Here's how the part is built. I have some questions about the finished solid (model axes, mm). Face numbers are marked on the shaded views. A direction names the side the tool comes from. Coordinates: 2 decimals unless noted, no trailing zeros. Write each loop counter-clockwise with the first axis right and the second up, starting at its lowest first coordinate (ties: lowest second). Pieces come first, ordered by that corner, then holes.
(1) Imagine slicing it at D-D, the plane y = 8. List the corners of the cut face in (x, z) for me.
(2) Imagine slicing it at B-B, the plane z = 40. State how many separate pieces and enclosed holes the cut face has, plus the area to 3 significant figures.
(3) Please list where these lines run through material, in increasing order: probe 1 along X at (y, z) = (18.55, 0); probe 2 along X at (y, z) = (17.95, 40); probe 3 along Y at (x, z) = (78, -41.5).
(4) Imagine slicing it at A-A, the plane x = 20.5. List the corners of the cut face in (y, z) for me, plus the area to 3 significant figures.
(5) Which directions (+Z, -Z, +X, -X, +Y, -Y) give clear straight access to the entire face, cutting with the end or side of a thin tool? Please do the marked faces 5 and 6.
(6) Thinking about a two-plate mould opening in Y: for the marked faces 1, 2, 3 and 4, which applies, released by +Y, released by -Y, zero draft, split by the parting line, or undercut?
(7) For pin 1 Ø2.5 at (x, z) = (4, -40) entering from -Y; pin 2 Ø1.9 at (x, z) = (30, -20.5) entering from +Y, each with a flat end and sliding along its axis, tell me the tip position at first contact or that it passes through.
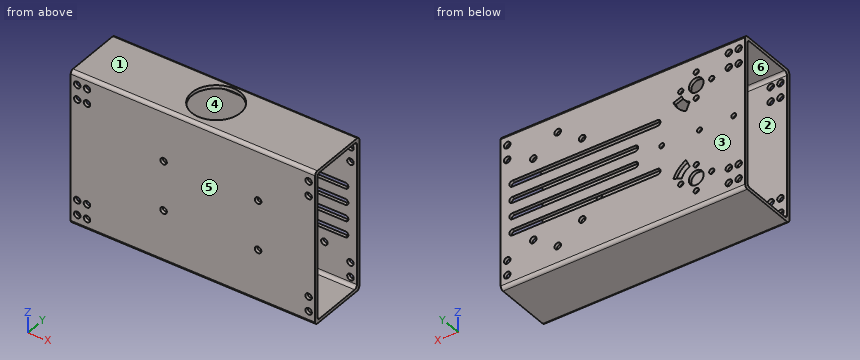
```python
from build123d import *

# Parameters (mm, degrees)
EXTRUDE_1218_DEPTH          = 150
SKETCH_1_R                  = 1.5
SKETCH_1_R_2                = 4.5
SKETCH_1_R_3                = 1.6
CUT_EXTRUDE_1265_DEPTH      = 159.33508771
SKETCH_6_R                  = 15
CUT_EXTRUDE_1532_DEPTH      = 159.33508771
SKETCH_12_R                 = 2
CUT_EXTRUDE_1963_DEPTH      = 2
CUT_EXTRUDE_2327_DEPTH      = 162.260658685
CUT_EXTRUDE_2327_DEPTH_BACK = 162.260658685
SKETCH_14_R                 = 2
SKETCH_15_R                 = 2
CUT_EXTRUDE_2529_DEPTH      = 162.260658685


with BuildPart() as part:
    # 草图2 → Extrude 1218 (new body)
    with BuildSketch(Plane(origin=(0, 0, 0), x_dir=(0, 0, -1), z_dir=(1, 0, 0))):
        with BuildLine():
            Line((-45, 19), (45, 19))
            ThreePointArc((45, 19), (46.414213562, 18.414213562), (47, 17))
            Line((47, 17), (47, -17))
            ThreePointArc((47, -17), (46.414213562, -18.414213562), (45, -19))
            Line((45, -19), (-45, -19))
            ThreePointArc((-45, -19), (-46.414213562, -18.414213562), (-47, -17))
            Line((-47, -17), (-47, 17))
            ThreePointArc((-47, 17), (-46.414213562, 18.414213562), (-45, 19))
        make_face()
        with BuildLine():
            Line((-43, 17), (43, 17))
            ThreePointArc((43, 17), (44.414213562, 16.414213562), (45, 15))
            Line((45, 15), (45, -15))
            ThreePointArc((45, -15), (44.414213562, -16.414213562), (43, -17))
            Line((43, -17), (-43, -17))
            ThreePointArc((-43, -17), (-44.414213562, -16.414213562), (-45, -15))
            Line((-45, -15), (-45, 15))
            ThreePointArc((-45, 15), (-44.414213562, 16.414213562), (-43, 17))
        make_face(mode=Mode.SUBTRACT)
    extrude(amount=EXTRUDE_1218_DEPTH)

    # 草图1 → Cut-Extrude 1265 (cut, through all)
    with BuildSketch(Plane(origin=(0, 0, 0), x_dir=(1, 0, 0), z_dir=(0, 1, 0))):
        with Locations(Location((7, 0, 0), (0, 0, 90))):
            Circle(SKETCH_1_R)
        with Locations(Location((28, 0, 0), (0, 0, 90))):
            Circle(SKETCH_1_R)
        with Locations(Location((51.2, 0, 0), (0, 0, 90))):
            Circle(SKETCH_1_R)
        with Locations(Location((30, -28.5, 0), (0, 0, 90))):
            Circle(SKETCH_1_R_2)
        with Locations(Location((30, 28.5, 0), (0, 0, 90))):
            Circle(SKETCH_1_R_2)
        with Locations(Location((20.5, -28.5, 0), (0, 0, 90))):
            Circle(SKETCH_1_R_3)
        with Locations(Location((39.5, -28.5, 0), (0, 0, 90))):
            Circle(SKETCH_1_R_3)
        with Locations(Location((30, -36.5, 0), (0, 0, 90))):
            Circle(SKETCH_1_R_3)
        with Locations(Location((30, -20.5, 0), (0, 0, 90))):
            Circle(SKETCH_1_R_3)
        with Locations(Location((39.5, 28.5, 0), (0, 0, 90))):
            Circle(SKETCH_1_R_3)
        with Locations(Location((30, 36.5, 0), (0, 0, 90))):
            Circle(SKETCH_1_R_3)
        with Locations(Location((20.5, 28.5, 0), (0, 0, 90))):
            Circle(SKETCH_1_R_3)
        with Locations(Location((30, 20.5, 0), (0, 0, 90))):
            Circle(SKETCH_1_R_3)
        with BuildLine():
            Line((34.014873487, 19.890076023), (36.291936994, 15.006897573))
            ThreePointArc((36.291936994, 15.006897573), (40.941044845, 18.474379532), (43.990135541, 23.40800709))
            Line((43.990135541, 23.40800709), (38.927079897, 25.250808638))
            ThreePointArc((38.927079897, 25.250808638), (37.0041347, 22.081893028), (34.014873487, 19.890076023))
        make_face()
        with BuildLine():
            Line((34.014873487, -19.890076023), (36.291936994, -15.006897573))
            ThreePointArc((36.291936994, -15.006897573), (40.941044845, -18.474379532), (43.990135541, -23.40800709))
            Line((43.990135541, -23.40800709), (38.927079897, -25.250808638))
            ThreePointArc((38.927079897, -25.250808638), (37.0041347, -22.081893028), (34.014873487, -19.890076023))
        make_face()
    extrude(amount=CUT_EXTRUDE_1265_DEPTH, mode=Mode.SUBTRACT)

    # 草图6 → Cut-Extrude 1532 (cut, through all)
    with BuildSketch(Plane.XY):
        with Locations(Location((75, 1, 0), (0, 0, 111.039469781))):
            Circle(SKETCH_6_R)
    extrude(amount=CUT_EXTRUDE_1532_DEPTH, mode=Mode.SUBTRACT)

    # 草图12 → Cut-Extrude 1963 (cut)
    with BuildSketch(Plane(origin=(0, 19, 0), x_dir=(1, 0, 0), z_dir=(0, 1, 0))):
        with Locations(Location((100, 25, 0), (0, 0, 270))):
            Circle(SKETCH_12_R)
        with Locations(Location((130, 25, 0), (0, 0, 270))):
            Circle(SKETCH_12_R)
        with Locations(Location((115, 35, 0), (0, 0, 270))):
            Circle(SKETCH_12_R)
        with Locations(Location((115, -35, 0), (0, 0, 90))):
            Circle(SKETCH_12_R)
        with Locations(Location((130, -25, 0), (0, 0, 90))):
            Circle(SKETCH_12_R)
        with Locations(Location((100, -25, 0), (0, 0, 90))):
            Circle(SKETCH_12_R)
        with BuildLine():
            Line((53.777197841, 16.849529373), (142.85706065, 16.849529373))
            ThreePointArc((142.85706065, 16.849529373), (144.706590023, 15), (142.85706065, 13.150470627))
            Line((142.85706065, 13.150470627), (53.777197841, 13.150470627))
            ThreePointArc((53.777197841, 13.150470627), (51.927668468, 15), (53.777197841, 16.849529373))
        make_face()
        with BuildLine():
            Line((67.529255568, 6.850912176), (142.85706065, 6.850912176))
            ThreePointArc((142.85706065, 6.850912176), (144.707972825, 5), (142.85706065, 3.149087824))
            Line((142.85706065, 3.149087824), (67.529255568, 3.149087824))
            ThreePointArc((67.529255568, 3.149087824), (65.678343393, 5), (67.529255568, 6.850912176))
        make_face()
        with BuildLine():
            Line((53.777197841, -16.849529373), (142.85706065, -16.849529373))
            ThreePointArc((142.85706065, -16.849529373), (144.706590023, -15), (142.85706065, -13.150470627))
            Line((142.85706065, -13.150470627), (53.777197841, -13.150470627))
            ThreePointArc((53.777197841, -13.150470627), (51.927668468, -15), (53.777197841, -16.849529373))
        make_face()
        with BuildLine():
            Line((67.529255568, -6.850912176), (142.85706065, -6.850912176))
            ThreePointArc((142.85706065, -6.850912176), (144.707972825, -5), (142.85706065, -3.149087824))
            Line((142.85706065, -3.149087824), (67.529255568, -3.149087824))
            ThreePointArc((67.529255568, -3.149087824), (65.678343393, -5), (67.529255568, -6.850912176))
        make_face()
    extrude(amount=-CUT_EXTRUDE_1963_DEPTH, mode=Mode.SUBTRACT)

    # 草图14 → Cut-Extrude 2327 (cut, two sides: drawn at the far end of the back side and taken through both)
    with BuildSketch(Plane(origin=(0, -17, 0), x_dir=(1, 0, 0), z_dir=(0, 1, 0)).offset(-CUT_EXTRUDE_2327_DEPTH_BACK)):
        with Locations(Location((4, 40, 0), (0, 0, 270))):
            Circle(SKETCH_14_R)
        with Locations(Location((4, 31, 0), (0, 0, 270))):
            Circle(SKETCH_14_R)
        with Locations(Location((4, -31, 0), (0, 0, 90))):
            Circle(SKETCH_14_R)
        with Locations(Location((4, -40, 0), (0, 0, 90))):
            Circle(SKETCH_14_R)
        with Locations(Location((146, 40, 0), (0, 0, 270))):
            Circle(SKETCH_14_R)
        with Locations(Location((146, 31, 0), (0, 0, 270))):
            Circle(SKETCH_14_R)
        with Locations(Location((146, -40, 0), (0, 0, 90))):
            Circle(SKETCH_14_R)
        with Locations(Location((146, -31, 0), (0, 0, 90))):
            Circle(SKETCH_14_R)
        with Locations(Location((10, 40, 0), (0, 0, 270))):
            Circle(SKETCH_14_R)
        with Locations(Location((10, 31, 0), (0, 0, 270))):
            Circle(SKETCH_14_R)
        with Locations(Location((10, -40, 0), (0, 0, 90))):
            Circle(SKETCH_14_R)
        with Locations(Location((10, -31, 0), (0, 0, 90))):
            Circle(SKETCH_14_R)
    extrude(amount=CUT_EXTRUDE_2327_DEPTH + CUT_EXTRUDE_2327_DEPTH_BACK, mode=Mode.SUBTRACT)

    # 草图15 → Cut-Extrude 2529 (cut, through all)
    with BuildSketch(Plane(origin=(0, -17, 0), x_dir=(1, 0, 0), z_dir=(0, 1, 0))):
        with Locations(Location((57, 15.150470627, 0), (0, 0, 270))):
            Circle(SKETCH_15_R)
        with Locations(Location((57, -15.150470627, 0), (0, 0, 270))):
            Circle(SKETCH_15_R)
        with Locations(Location((115, 15.150470627, 0), (0, 0, 270))):
            Circle(SKETCH_15_R)
        with Locations(Location((115, -15.150470627, 0), (0, 0, 270))):
            Circle(SKETCH_15_R)
    extrude(amount=-CUT_EXTRUDE_2529_DEPTH, mode=Mode.SUBTRACT)


solid = part.part
```
Recorded:
1. outline: (0, -47) - (150, -47) - (150, -45) - (0, -45) - close; (0, 45) - (61.73, 45) - (61.73, 47) - (0, 47) - close; (88.27, 45) - (150, 45) - (150, 47) - (88.27, 47) - close
2. separate pieces: 8
2. enclosed holes: 0
2. area: 552 mm2
3. probe 1: x = 0 to 5.5, 8.5 to 26.5, 29.5 to 49.7, 52.7 to 150
3. probe 2: x = 0 to 2, 6 to 8, 12 to 144, 148 to 150
3. probe 3: y = -19 to -17, 17 to 19
4. outline: (-19, -45) arc R2 ccw to (-17, -47) - (17, -47) arc R2 ccw to (19, -45) - (19, -30.1) - (17, -30.1) - (17, -43) arc R2 cw to (15, -45) - (-15, -45) arc R2 cw to (-17, -43) - (-17, 43) arc R2 cw to (-15, 45) - (15, 45) arc R2 cw to (17, 43) - (17, 30.1) - (19, 30.1) - (19, 45) arc R2 ccw to (17, 47) - (-17, 47) arc R2 ccw to (-19, 45) - close; (17, -26.9) - (19, -26.9) - (19, 26.9) - (17, 26.9) - close
4. area: 499 mm2
5. face 5: +Z, -Z, +X, -X, -Y
5. face 6: +X, -X
6. face 1: zero draft
6. face 2: undercut
6. face 3: released by +Y
6. face 4: undercut
7. pin 1: passes through
7. pin 2: stops at y = -17
